```python
from build123d import *

# Parameters (mm, degrees)
F1_DEPTH       = 3
F3_D           = 4.2
F3_CSINK_D     = 7.5
F3_CSINK_ANGLE = 90
F4_T1_DEPTH    = 5.2623442452


# Not quite as in the source:
# - a fillet or chamfer that OpenCascade refuses, or shapes differently, is made with other operations: its cross-section is extruded or revolved along the edge and cut away or added


with BuildPart() as f1:
    # F0 (on Front) → F1 (new body)
    with BuildSketch(Plane.XZ):
        with BuildLine():
            Line((-13, 0), (0, 0))
            Line((0, 0), (0, 10))
            Line((0, 10), (-9, 10))
            Line((-9, 10), (-9, 5.5))
            ThreePointArc((-9, 5.5), (-10.5, 4), (-12, 5.5))
            Line((-12, 5.5), (-13, 5.5))
            Line((-13, 5.5), (-13, 0))
        make_face()
    extrude(amount=-F1_DEPTH)

    # F3 (through all)
    with Locations(Plane.XZ):
        with Locations((-4.5, 5)):
            CounterSinkHole(F3_D / 2, F3_CSINK_D / 2, counter_sink_angle=F3_CSINK_ANGLE)

    # F4: chamfer of 0.5 on 1 edges, made by hand

    # F4_s2 → F4_t1 (cut)
    with BuildSketch(Plane.XZ.offset(-4.1311721226)):
        with BuildLine():
            Line((-12.4364916731, 5.5), (-11.9523687548, 5.125))
            ThreePointArc((-11.9523687548, 5.125), (-11.9871251619, 5.3038909672), (-12, 5.5))
            Line((-12, 5.5), (-12.4364916731, 5.5))
        make_face()
    extrude(amount=F4_T1_DEPTH, mode=Mode.SUBTRACT)


solid = f1.part
```
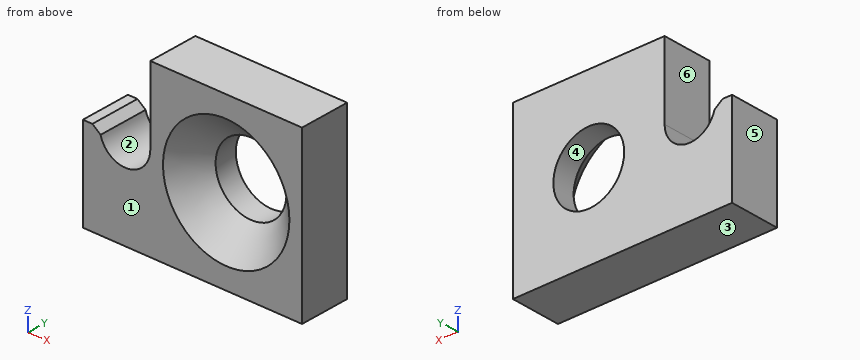
Work out the finished part from the listing and answer in its coordinate system (mm). Face numbers are marked on the shaded views. A direction names the side the tool comes from. Coordinates: 2 decimals unless noted, no trailing zeros. Loops run counter-clockwise (first coordinate to the right, second up) from the corner with the lowest first, then second, coordinate; pieces in that order, holes last. Notation, with made-up numbers: (-20.75, 73.25) - (30.25, 73.25) arc R38 cw to (30.25, 112.25) - close; hole circle Ø7 at (-35, -9). An arc over 180 degrees is marked (long way). Use a Markdown table: item, result.
Item 1: Consider probe 1 along Z at (x, y) = (-4.5, 2.45); probe 2 along X at (y, z) = (1.7, 4.75); probe 3 along X at (y, z) = (2.7, 5). Determine where each line is inside the solid, lowest interval first. Write a range as from..to.
Evaluation:
| item | result |
|---|---|
| probe 1 | z = 0..2.9, 7.1..10 |
| probe 2 | x = -13..-11.8, -9.2..-6.59, -2.41..0 |
| probe 3 | x = -13..-11.91, -9.09..-6.6, -2.4..0 |
Item 2: Find section C-C, the plane y = 2.05. Determine the outline of the cut face in (x, z) (1 decimal), and give its area (3 significant figures).
Evaluation:
| item | result |
|---|---|
| outline | (-13, 0) - (0, 0) - (0, 10) - (-9, 10) - (-9, 5.5) arc R1.5 cw to (-12, 5.1) - (-12.4, 5.5) - (-13, 5.5) - close; hole circle Ø4.2 at (-4.5, 5) |
| area | 94.5 mm2 |
Item 3: Find section B-B, the plane x = -4.5. Determine the outline of the cut face in (y, z).
Evaluation:
| item | result |
|---|---|
| outline | (0, 0) - (3, 0) - (3, 2.9) - (1.65, 2.9) - (0, 1.25) - close; (0, 8.75) - (1.65, 7.1) - (3, 7.1) - (3, 10) - (0, 10) - close |
Item 4: The mould has two halves that part along Z. Classify the marked faces 1, 2, 3 and 4: +Z half, -Z half, draft (parallel to the pull), parting line (faces both ways), or undercut.
Evaluation:
| item | result |
|---|---|
| face 1 | draft |
| face 2 | +Z half |
| face 3 | -Z half |
| face 4 | undercut |
Item 5: Given pin 1 Ø3.5 at (x, z) = (-4.5, 5) entering from -Y, flat-ended and moving along its own axis, determine where the tip first touches the part or whether it passes through.
Evaluation:
| item | result |
|---|---|
| pin 1 | passes through |
Item 6: Find section D-D, the plane x = -11.5. Determine the outline of the cut face in (y, z), and give its area (3 significant figures).
Evaluation:
| item | result |
|---|---|
| outline | (0, 0) - (3, 0) - (3, 4.38) - (0, 4.38) - close |
| area | 13.1 mm2 |
Item 7: For the marked faces 5 and 6, determine the directions among +Z, -Z, +X, -X, +Y, -Y from which every point of the face is accessible in a straight line to the end or side of a thin tool.
Evaluation:
| item | result |
|---|---|
| face 5 | +Z, -Z, -X, +Y, -Y |
| face 6 | +Z, -X, +Y, -Y |
